```python
from build123d import *

# Parameters (mm, degrees)
SKETCH1_R                           = 18
BOSS_EXTRUDE1_DEPTH                 = 56
FILLET1_R                           = 3
CUT_EXTRUDE1_START                  = -14.96663
CUT_EXTRUDE1_DEPTH                  = 29.93326
SKETCH3_W                           = 13
SKETCH3_H                           = 1
SKETCH4_R                           = 5.5
BOSS_EXTRUDE2_DEPTH                 = 3
FILLET2_R                           = 0.5
SKETCH5_R                           = 1.5
BOSS_EXTRUDE3_DEPTH                 = 11
CUT_EXTRUDE2_REACH                  = 76.485
CUT_EXTRUDE2_END_RADIUS             = 1.5
SKETCH6_W                           = 9
SKETCH6_H                           = 0.5
CUT_EXTRUDE2_DIRECTION_2_REACH      = 76.485
CUT_EXTRUDE2_DIRECTION_2_END_RADIUS = 1.5
SKETCH7_R                           = 1.5
CUT_EXTRUDE3_DEPTH                  = 3


with BuildPart() as part:
    # Sketch1 → Boss-Extrude1 (new body)
    with BuildSketch(Plane(origin=(0, 0, 0), x_dir=(0, 0, -1), z_dir=(1, 0, 0))):
        Circle(SKETCH1_R)
    extrude(amount=BOSS_EXTRUDE1_DEPTH)

    # Fillet1
    fillet1_edges = [part.edges().sort_by_distance(p)[0] for p in [
        (56, 0, 18),
    ]]
    fillet(fillet1_edges, radius=FILLET1_R)

    # Sketch2 → Cut-Extrude1 (cut)
    with BuildSketch(Plane.XY.offset(CUT_EXTRUDE1_START)):
        Polygon((13, 18), (0, 10), (0, -10), (13, -18), (0, -18), (-7.803780753, 17.225837115), (0, 18), align=None)
    extrude(amount=CUT_EXTRUDE1_DEPTH, mode=Mode.SUBTRACT)

    # Sketch3 → Cut-Revolve1 (revolve, cut)
    with BuildSketch(Plane.XY, mode=Mode.PRIVATE) as cut_revolve1_sk:
        with Locations((6.5, 17.5)):
            Rectangle(SKETCH3_W, SKETCH3_H)
    revolve(cut_revolve1_sk.sketch.rotate(Axis((-1000, 0, 0), (1, 0, 0)), 90), axis=Axis((-1000, 0, 0), (1, 0, 0)), mode=Mode.SUBTRACT)

    # Sketch4 → Boss-Extrude2 (add)
    with BuildSketch(Plane(origin=(56, 0, 0), x_dir=(0, 0, -1), z_dir=(1, 0, 0))):
        Circle(SKETCH4_R)
    extrude(amount=BOSS_EXTRUDE2_DEPTH)

    # Fillet2
    fillet2_edges = [part.edges().sort_by_distance(p)[0] for p in [
        (59, 0, 5.5),
    ]]
    fillet(fillet2_edges, radius=FILLET2_R)

    # Sketch5 → Boss-Extrude3 (add)
    with BuildSketch(Plane(origin=(59, 0, 0), x_dir=(0, 0, -1), z_dir=(1, 0, 0))):
        Circle(SKETCH5_R)
    extrude(amount=BOSS_EXTRUDE3_DEPTH)

    # Cut-Extrude2: up to this cylinder (the profile starts inside it)
    cut_extrude2_end = Plane(origin=(65.5, 0, 0), z_dir=(-1, 0, 0)) * Cylinder(CUT_EXTRUDE2_END_RADIUS, 156.97, mode=Mode.PRIVATE)
    # Sketch6 → Cut-Extrude2 (cut, up to the surface)
    with BuildSketch(Plane.XY, mode=Mode.PRIVATE) as cut_extrude2_sk1:
        with Locations((65.5, 1.25)):
            Rectangle(SKETCH6_W, SKETCH6_H)
    cut_extrude2_tool1 = extrude(cut_extrude2_sk1.sketch, amount=-CUT_EXTRUDE2_REACH, mode=Mode.PRIVATE) & cut_extrude2_end
    add(cut_extrude2_tool1.solids().sort_by_distance((65.5, 1.25, 0))[0], mode=Mode.SUBTRACT)

    # Cut-Extrude2 direction 2: up to this cylinder (the profile starts inside it)
    cut_extrude2_direction_2_end = Plane(origin=(65.5, 0, 0), z_dir=(-1, 0, 0)) * Cylinder(CUT_EXTRUDE2_DIRECTION_2_END_RADIUS, 156.97, mode=Mode.PRIVATE)
    # Sketch6 → Cut-Extrude2 direction 2 (cut, up to the surface)
    with BuildSketch(Plane.XY, mode=Mode.PRIVATE) as cut_extrude2_direction_2_sk1:
        with Locations((65.5, 1.25)):
            Rectangle(SKETCH6_W, SKETCH6_H)
    cut_extrude2_direction_2_tool1 = extrude(cut_extrude2_direction_2_sk1.sketch, amount=CUT_EXTRUDE2_DIRECTION_2_REACH, mode=Mode.PRIVATE) & cut_extrude2_direction_2_end
    add(cut_extrude2_direction_2_tool1.solids().sort_by_distance((65.5, 1.25, 0))[0], mode=Mode.SUBTRACT)

    # Sketch7 → Cut-Extrude3 (cut)
    with BuildSketch(Plane(origin=(56, 0, 0), x_dir=(0, 0, -1), z_dir=(1, 0, 0))):
        with Locations((0, 12.5)):
            Circle(SKETCH7_R)
        with Locations((12.5, 0)):
            Circle(SKETCH7_R)
        with Locations((0, -12.5)):
            Circle(SKETCH7_R)
        with Locations((-12.5, 0)):
            Circle(SKETCH7_R)
    extrude(amount=-CUT_EXTRUDE3_DEPTH, mode=Mode.SUBTRACT)


solid = part.part
```
Source: CAD feature listing. Evaluate the final solid. Frame: model axes, mm. A direction names the side the tool comes from. Round coordinates to 2 decimals unless told otherwise and drop trailing zeros. Order: outer loops, then holes, each group sorted by start corner. A loop starts at its lowest first (then second) coordinate and runs counter-clockwise, first axis right, second up. Notation, with made-up numbers: (25, 42) -> (63, 42) arc R31 cw to (63, 77) -> close; hole circle Ø7 at (44, 29.5). An arc over 180 degrees is marked (long way). One line per item, written item: value. Start each with the question number.
Q1. Access query for faces 1 (the flat face through (65, 1, 0)), 2 (the flat face through (53, 0, -12)), 3 (the flat face through (13, 16, -7)). Directions: +Z, -Z, +X, -X, +Y, -Y. A direction counts if a zero-diameter tool reaches every point of the face in a straight line with its end or side. Return the directions, or none.
Q2. Section query B-B (y = 0). Return the cut outline in (x, z), plus the area to 3 significant figures.
Q3. Section query C-C (x = 54.5). Return the cut outline in (y, z), plus the area to 3 significant figures.
Q4. Pin query (flat end, axial travel): pin 1 (4 mm diameter, centred on x = 38.5, y = -9.5, fed in from -Z); pin 2 (1.1 mm diameter, centred on x = 67.5, z = 0, fed in from +Y); pin 3 (10 mm diameter, centred on x = 12, z = 6, fed in from -Y). Return the tip coordinate at first contact, or that it passes through.
Q5. Material intervals for probe 1 along X at (y, z) = (0, -6); probe 2 along Z at (x, y) = (32, 0.5); probe 3 along Y at (x, z) = (54, 0), sorted ascending.
Q6. Section query D-D (x = 33). Return the cut outline in (y, z).
Findings below:
1. face 1: +Z, -Z, +X, +Y
1. face 2: +X
1. face 3: -X
2. outline: (0, -17) -> (13, -17) -> (13, -18) -> (53, -18) arc R3 ccw to (56, -15) -> (56, -14) -> (53, -14) -> (53, -11) -> (56, -11) -> (56, -5.5) -> (58.5, -5.5) arc R0.5 ccw to (59, -5) -> (59, -1.5) -> (70, -1.5) -> (70, 1.5) -> (59, 1.5) -> (59, 5) arc R0.5 ccw to (58.5, 5.5) -> (56, 5.5) -> (56, 11) -> (53, 11) -> (53, 14) -> (56, 14) -> (56, 15) arc R3 ccw to (53, 18) -> (13, 18) -> (13, 17) -> (0, 17) -> close
2. area: 2,030 mm²
3. outline: circle Ø35.2 at (0, 0); hole circle Ø3 at (-12.5, 0); hole circle Ø3 at (0, -12.5); hole circle Ø3 at (0, 12.5); hole circle Ø3 at (12.5, 0)
3. area: 945 mm²
4. pin 1: z = -16.36
4. pin 2: y = 1
4. pin 3: y = -17.97
5. probe 1: 0 to 56
5. probe 2: -17.99 to 17.99
5. probe 3: -17.83 to -14, -11 to 11, 14 to 17.83
6. outline: circle Ø36 at (0, 0)
